```python
from build123d import *

# Parameters (mm, degrees)
SKETCH1_R           = 16.764
SKETCH1_R_2         = 13.335
BOSS_EXTRUDE1_DEPTH = 12.7
SKETCH2_W           = 54.028772228
SKETCH2_H           = 66.192828526
BOSS_EXTRUDE2_DEPTH = 152.4
FILLET1_R           = 7.62
FILLET2_R           = 12.7
FILLET3_R           = 12.7
FILLET4_R           = 7.62
BOSS_EXTRUDE3_START = 12.7
SKETCH3_R           = 16.764
SKETCH3_R_2         = 13.335
BOSS_EXTRUDE3_DEPTH = 12.7
SKETCH4_R           = 16.764
SKETCH4_R_2         = 13.335
BOSS_EXTRUDE4_DEPTH = 12.7
BOSS_EXTRUDE5_DEPTH = 2.54


with BuildPart() as part:
    # Sketch1 → Boss-Extrude1 (new body)
    with BuildSketch(Plane(origin=(0, 0, 0), x_dir=(0, 0, -1), z_dir=(1, 0, 0))):
        Circle(SKETCH1_R)
        Circle(SKETCH1_R_2, mode=Mode.SUBTRACT)
    extrude(amount=BOSS_EXTRUDE1_DEPTH)

    # Sketch2 → Boss-Extrude2 (add)
    with BuildSketch(Plane.ZY):
        Rectangle(SKETCH2_W, SKETCH2_H)
    extrude(amount=BOSS_EXTRUDE2_DEPTH)

    # Fillet1
    fillet1_edges = [part.edges().sort_by_distance(p)[0] for p in [
        (0, 33.096414263, 0),
        (0, 0, -27.014386114),
        (0, -33.096414263, 0),
        (0, 0, 27.014386114),
    ]]
    fillet(fillet1_edges, radius=FILLET1_R)

    # Fillet2
    # the kernel refuses this fillet: 12.7 mm, written as the material it takes off along each edge
    with BuildSketch(Plane(origin=(0, -20.396414263, -14.314386114), x_dir=(0, -1, 0), z_dir=(0, 0, 1))) as fillet2_piece_1:
        with BuildLine():
            CenterArc((5.08, -7.62), 7.62, 0, 90)
            Line((12.7, -7.62), (12.7, 0))
            Line((12.7, 0), (5.08, 0))
        make_face()
    revolve(axis=Axis((0, -20.396414263, -14.314386114), (1, 0, 0)), revolution_arc=90, mode=Mode.SUBTRACT)
    with BuildSketch(Plane(origin=(0, 20.396414263, -14.314386114), x_dir=(0, 0, -1), z_dir=(0, -1, 0))) as fillet2_piece_2:
        with BuildLine():
            CenterArc((5.08, -7.62), 7.62, 0, 90)
            Line((12.7, -7.62), (12.7, 0))
            Line((12.7, 0), (5.08, 0))
        make_face()
    revolve(axis=Axis((0, 20.396414263, -14.314386114), (1, 0, 0)), revolution_arc=90, mode=Mode.SUBTRACT)
    with BuildSketch(Plane(origin=(0, 20.396414263, 14.314386114), x_dir=(0, 1, 0), z_dir=(0, 0, -1))) as fillet2_piece_3:
        with BuildLine():
            CenterArc((5.08, -7.62), 7.62, 0, 90)
            Line((12.7, -7.62), (12.7, 0))
            Line((12.7, 0), (5.08, 0))
        make_face()
    revolve(axis=Axis((0, 20.396414263, 14.314386114), (1, 0, 0)), revolution_arc=90, mode=Mode.SUBTRACT)
    with BuildSketch(Plane(origin=(0, 33.096414263, 27.014386114), x_dir=(0, -1, 0), z_dir=(-1, 0, 0))) as fillet2_piece_4:
        with BuildLine():
            CenterArc((FILLET2_R, -FILLET2_R), FILLET2_R, 90, 90)
            Line((0, -FILLET2_R), (0, 0))
            Line((0, 0), (FILLET2_R, 0))
        make_face()
    extrude(amount=184.15, mode=Mode.SUBTRACT)
    with BuildSketch(Plane(origin=(0, 33.096414263, -27.014386114), x_dir=(0, -1, 0), z_dir=(-1, 0, 0)), Plane(origin=(0, -33.096414263, -27.014386114), x_dir=(0, 0, 1), z_dir=(-1, 0, 0))) as fillet2_piece_5:
        with BuildLine():
            CenterArc((FILLET2_R, FILLET2_R), FILLET2_R, 180, 90)
            Line((0, FILLET2_R), (0, 0))
            Line((0, 0), (FILLET2_R, 0))
        make_face()
    extrude(amount=184.15, mode=Mode.SUBTRACT)

    # Fillet3
    # the kernel refuses this fillet: 12.7 mm, written as the material it takes off along each edge
    with BuildSketch(Plane(origin=(0, -20.396414263, 14.314386114), x_dir=(0, 0, 1), z_dir=(0, 1, 0))) as fillet3_piece_1:
        with BuildLine():
            CenterArc((5.08, -7.62), 7.62, 0, 90)
            Line((12.7, -7.62), (12.7, 0))
            Line((12.7, 0), (5.08, 0))
        make_face()
    revolve(axis=Axis((0, -20.396414263, 14.314386114), (1, 0, 0)), revolution_arc=90, mode=Mode.SUBTRACT)
    with BuildSketch(Plane(origin=(0, -33.096414263, 27.014386114), x_dir=(0, 0, -1), z_dir=(-1, 0, 0))) as fillet3_piece_2:
        with BuildLine():
            CenterArc((FILLET3_R, -FILLET3_R), FILLET3_R, 90, 90)
            Line((0, -FILLET3_R), (0, 0))
            Line((0, 0), (FILLET3_R, 0))
        make_face()
    extrude(amount=184.15, mode=Mode.SUBTRACT)

    # Fillet4
    fillet4_edges = [part.edges().sort_by_distance(p)[0] for p in [
        (-152.4, -33.096414263, 0),
        (-152.4, 0, -27.014386114),
        (-152.4, 33.096414263, 0),
        (-152.4, 29.376670384, -23.294642235),
        (-152.4, 29.376670384, 23.294642235),
        (-152.4, -29.376670384, -23.294642235),
        (-152.4, 0, 27.014386114),
        (-152.4, -29.376670384, 23.294642235),
    ]]
    fillet(fillet4_edges, radius=FILLET4_R)

    # Sketch3 → Boss-Extrude3 (add)
    with BuildSketch(Plane.ZY.offset(152.4).offset(BOSS_EXTRUDE3_START)):
        with Locations(Location((0, 0, 0), (0, 0, 180))):
            Circle(SKETCH3_R)
        with Locations(Location((0, 0, 0), (0, 0, 180))):
            Circle(SKETCH3_R_2, mode=Mode.SUBTRACT)
    extrude(amount=-BOSS_EXTRUDE3_DEPTH)

    # Sketch4 → Boss-Extrude4 (add)
    with BuildSketch(Plane.XZ.offset(33.096414263)):
        with Locations(Location((-123.986445469, 0, 0), (0, 0, 58.635839184))):
            Circle(SKETCH4_R)
        with Locations(Location((-123.986445469, 0, 0), (0, 0, 270))):
            Circle(SKETCH4_R_2, mode=Mode.SUBTRACT)
    extrude(amount=BOSS_EXTRUDE4_DEPTH)

    # Sketch5 → Boss-Extrude5 (add)
    with BuildSketch(Plane(origin=(0, 0, -27.014386114), x_dir=(-1, 0, 0), z_dir=(0, 0, -1))):
        Polygon((53.996659103, 0), (87.835708054, 0), (87.835708054, 6.35), (96.484197887, -3.175), (87.835708054, -12.7), (87.835708054, -6.35), (53.996659103, -6.35), align=None)
    extrude(amount=BOSS_EXTRUDE5_DEPTH)


solid = part.part
```
For this review, take the finished solid that the model builds, in its own axes (mm). A direction names the side the tool comes from. Round coordinates to 2 decimals unless told otherwise and drop trailing zeros. Write each loop counter-clockwise with the first axis right and the second up, starting at its lowest first coordinate (ties: lowest second). Pieces come first, ordered by that corner, then holes.
1) Insertion check: pin 1 Ø4 at (x, z) = (-90, 1) entering from -Y; pin 2 Ø13.5 at (y, z) = (1.5, -5.5) entering from -X; pin 3 Ø1.3 at (y, z) = (2.5, -28) entering from +X. Each pin has a flat end and moves straight along its axis. Give the tip position at first contact, or say it passes through.
Answer below:
pin 1: stops at y = -33.1
pin 2: stops at x = -152.4
pin 3: stops at x = -87.84
2) Mouldability with a two-part tool opening along Z and no side actions: class faces 6 (the face through (-152.4, 0, 0)), 7 (the face through (6, 5, -16)), 8 (the face through (-110.765, -39.358, 1.736)), 9 (the face through (-75, 33.096, 0)) as +Z half, -Z half, draft (parallel to the pull), parting line (faces both ways), or undercut.
Answer below:
face 6: undercut
face 7: parting line
face 8: undercut
face 9: draft
3) Take a section at A-A on x = -40. Give the boundary of the cut face in (y, z).
Answer below:
outline: (-33.1, -14.31) arc R12.7 ccw to (-20.4, -27.01) - (20.4, -27.01) arc R12.7 ccw to (33.1, -14.31) - (33.1, 14.31) arc R12.7 ccw to (20.4, 27.01) - (-20.4, 27.01) arc R12.7 ccw to (-33.1, 14.31) - close
4) Take a section at C-C on y = -11. Give the boundary of the cut face in (x, z), then the cut area to 3 significant figures.
Answer below:
outline: (-165.1, -12.65) - (-152.4, -12.65) - (-152.4, -19.39) arc R7.62 ccw to (-144.78, -27.01) - (-89.38, -27.01) - (-89.38, -29.55) - (-87.84, -29.55) - (-87.84, -27.01) - (-7.62, -27.01) arc R7.62 ccw to (0, -19.39) - (0, -12.65) - (12.7, -12.65) - (12.7, -7.54) - (0, -7.54) - (0, 7.54) - (12.7, 7.54) - (12.7, 12.65) - (0, 12.65) - (0, 19.39) arc R7.62 ccw to (-7.62, 27.01) - (-144.78, 27.01) arc R7.62 ccw to (-152.4, 19.39) - (-152.4, 12.65) - (-165.1, 12.65) - (-165.1, 7.54) - (-152.4, 7.54) - (-152.4, -7.54) - (-165.1, -7.54) - close
area: 8,450 mm2
5) For line 1 along Y through (x, z) = (10, 0) (3 decimals); line 2 along X through (y, z) = (-13.5, -20); line 3 along Y through (x, z) = (-17.5, 13), list the stretches that pass through material, from the lowest coordinate up.
Answer below:
line 1: y = -16.764 to -13.335, 13.335 to 16.764
line 2: x = -152.38 to -0.02
line 3: y = -33.1 to 33.1
6) Take a section at D-D on x = -79.5. Give the boundary of the cut face in (y, z).
Answer below:
outline: (-33.1, -14.31) arc R12.7 ccw to (-20.4, -27.01) - (-6.35, -27.01) - (-6.35, -29.55) - (0, -29.55) - (0, -27.01) - (20.4, -27.01) arc R12.7 ccw to (33.1, -14.31) - (33.1, 14.31) arc R12.7 ccw to (20.4, 27.01) - (-20.4, 27.01) arc R12.7 ccw to (-33.1, 14.31) - close
7) Machinability: for faces 1 (the face through (-2.29, -30.92, 0.2)), 2 (the face through (-92.099, 1.654, -28.267)), 3 (the face through (0, 17, 0)), 4 (the face through (-141, -33.096, 0)), 5 (the face through (12.7, -7.4, 11.3)), which of the approach directions +Z, -Z, +X, -X, +Y, -Y give a long, thin tool a straight path to every point of the face, cutting with its end or side? Answer none if there is none.
Answer below:
face 1: +Z, -Z, +X, -Y
face 2: -Z, -X, +Y
face 3: +X
face 4: -X, -Y
face 5: +Z, -Z, +X, +Y, -Y
